```python
from build123d import *

# Parameters (mm, degrees)
F2_W      = 90
F2_H      = 90
F6_W      = 82
F6_H      = 82
F12_DEPTH = 5
F13_DEPTH = 10.1
F14_DEPTH = 10
F15_DEPTH = 10
F16_W     = 1.180001
F16_H     = 1.870001
F16_W_2   = 1.18
F16_H_2   = 4.060001
F16_W_3   = 10.110001
F16_H_3   = 1.18
F16_W_4   = 6.670001
F17_DEPTH = 2


# Not quite as in the source:
# - the dataset's text gives a spline's control points without its knots; the knots are read off the source's solid


with BuildPart() as f3:
    # F2 (on Top) → F3 section 0
    with BuildSketch(Plane.XY, mode=Mode.PRIVATE) as f3_s0:
        Rectangle(F2_W, F2_H)
    loft([f3_s0.sketch, Vertex(0, 0, 63.6368)])

    # F6 (on face) → F7 section 0
    with BuildSketch(Plane.XY, mode=Mode.PRIVATE) as f7_s0:
        Rectangle(F6_W, F6_H)
    loft([f7_s0.sketch, Vertex(0, 0, 58.6368)], mode=Mode.SUBTRACT)

    # F8 (on face) → F12 (cut, symmetric)
    with BuildSketch(Plane(origin=(29.9991167733, 0, 21.2135156827), x_dir=(0, 1, 0), z_dir=(0.8164845616, 0, 0.5773672666))):
        Polygon((0.1463476627, 39.9593571873), (-28.0024763197, -8.9000007138), (27.9615262598, -8.9000007138), align=None)
    extrude(amount=F12_DEPTH, both=True, mode=Mode.SUBTRACT)

    # F9 (on face) → F13 (cut)
    with BuildSketch(Plane(origin=(0, 29.9991167733, 21.2135156827), x_dir=(-1, 0, 0), z_dir=(0, 0.8164845616, 0.5773672666))):
        Polygon((0.1463476627, 39.9593571873), (-27.835653627, -8.5054690465), (28.1283489525, -8.5054690465), align=None)
    extrude(amount=-F13_DEPTH, mode=Mode.SUBTRACT)

    # F10 (on face) → F14 (cut)
    with BuildSketch(Plane(origin=(-29.9991167733, 0, 21.2135156827), x_dir=(0, -1, 0), z_dir=(-0.8164845616, 0, 0.5773672666))):
        Polygon((0.1463476627, 39.9593571873), (-28.9770383388, -9.5114903525), (26.9869642407, -9.5114903525), align=None)
    extrude(amount=-F14_DEPTH, mode=Mode.SUBTRACT)

    # F11 (on face) → F15 (cut)
    with BuildSketch(Plane(origin=(0, -29.9991167733, 21.2135156827), x_dir=(1, 0, 0), z_dir=(0, -0.8164845616, 0.5773672666))):
        Polygon((0.1463476627, 39.9593571873), (-28.0361250043, -9.3999961391), (27.9278775752, -9.3999961391), align=None)
    extrude(amount=-F15_DEPTH, mode=Mode.SUBTRACT)

    # F16 (on face) → F17 (cut)
    with BuildSketch(Plane(origin=(-29.9991167733, 0, 21.2135156827), x_dir=(0, -1, 0), z_dir=(-0.8164845616, 0, 0.5773672666))):
        Polygon((21.9697801374, -21.1938021154), (23.5597841374, -21.1938021154), (28.7397811374, -15.0950853876), (28.7397811374, -19.0038021154), (29.9197811374, -19.0038021154), (29.9197811374, -14.9538011154), (28.8597821374, -14.9538011154), (28.7397811374, -14.9538011154), (22.2197811374, -14.9538011154), (21.2197821374, -16.1338011154), (26.2597841374, -16.1338011154), align=None)
        with Locations((31.4797826374, -18.0688016154)):
            Rectangle(F16_W, F16_H)
        with Locations((33.6297791374, -19.1638016154)):
            Rectangle(F16_W_2, F16_H_2)
        Polygon((12.0897811374, -21.1938021154), (20.2597801374, -21.1938021154), (20.8297821374, -20.0438011154), (18.3297821374, -14.9538011154), (13.9597791374, -14.9538011154), (11.4997811374, -19.9838021154), align=None)
        Polygon((19.3697831374, -20.0138021154), (12.9197831374, -20.0138021154), (14.8197791374, -16.1338011154), (17.4797821374, -16.1338011154), align=None, mode=Mode.SUBTRACT)
        with BuildLine():
            Line((5.2997801374, -14.9538011154), (5.2997801374, -16.6038011154))
            add(Edge.make_bspline(
                [(4.1407171374, -16.7288011154), (4.3252931374, -16.7141861154), (4.7128221374, -16.6835011154), (5.0980381374, -16.6311951154), (5.2997801374, -16.6038011154)],
                knots=[0, 0, 0, 0, 0.555346, 1.165986, 1.165986, 1.165986, 1.165986], degree=3))
            add(Edge.make_bspline(
                [(3.2325931374, -16.7738011154), (3.3718421374, -16.7690131154), (3.6747741374, -16.7585981154), (3.9772701374, -16.7392531154), (4.1407171374, -16.7288011154)],
                knots=[0, 0, 0, 0, 0.417971, 0.909282, 0.909282, 0.909282, 0.909282], degree=3))
            add(Edge.make_bspline(
                [(2.4297801374, -16.7638011154), (2.5552081374, -16.7691171154), (2.8227031374, -16.7804551154), (3.0904121374, -16.7761091154), (3.2325931374, -16.7738011154)],
                knots=[0, 0, 0, 0, 0.376537, 0.803027, 0.803027, 0.803027, 0.803027], degree=3))
            Line((2.4297801374, -16.7638011154), (1.2497801374, -16.7638011154))
            Line((1.2497801374, -16.7638011154), (1.2497801374, -21.1938021154))
            Line((1.2497801374, -21.1938021154), (10.6597801374, -21.1938021154))
            Line((10.6597801374, -21.1938021154), (10.6597801374, -20.0138021154))
            Line((10.6597801374, -20.0138021154), (6.4797801374, -20.0138021154))
            Line((6.4797801374, -20.0138021154), (6.4797801374, -17.6491141154))
            add(Edge.make_bspline(
                [(8.6047791374, -17.0530201154), (8.2523501374, -17.1763541154), (7.5565571374, -17.4198491154), (6.8355751374, -17.5733591154), (6.4797801374, -17.6491141154)],
                knots=[0, 0, 0, 0, 1.118887, 2.208999, 2.208999, 2.208999, 2.208999], degree=3))
            add(Edge.make_bspline(
                [(10.6597801374, -16.1361451154), (10.3259741374, -16.3048751154), (9.6557671374, -16.6436461154), (8.9560111374, -16.9162101154), (8.6047791374, -17.0530201154)],
                knots=[0, 0, 0, 0, 1.121359, 2.251432, 2.251432, 2.251432, 2.251432], degree=3))
            Line((10.6597801374, -16.1361451154), (10.6597801374, -14.9538011154))
            add(Edge.make_bspline(
                [(8.5247801374, -15.8638011154), (8.8834781374, -15.7390181154), (9.6157961374, -15.4842611154), (10.3070901374, -15.1330071154), (10.6597801374, -14.9538011154)],
                knots=[0, 0, 0, 0, 1.137935, 2.323212, 2.323212, 2.323212, 2.323212], degree=3))
            add(Edge.make_bspline(
                [(6.4797801374, -16.4038011154), (6.8146711374, -16.3298001154), (7.5036441374, -16.1775551154), (8.1781381374, -15.9703101154), (8.5247801374, -15.8638011154)],
                knots=[0, 0, 0, 0, 1.028459, 2.115858, 2.115858, 2.115858, 2.115858], degree=3))
            Line((6.4797801374, -16.4038011154), (6.4797801374, -14.9538011154))
            Line((6.4797801374, -14.9538011154), (5.2997801374, -14.9538011154))
        make_face()
        with BuildLine():
            Line((5.2997801374, -20.0138021154), (2.4297801374, -20.0138021154))
            Line((2.4297801374, -20.0138021154), (2.4297801374, -17.9538021154))
            add(Edge.make_bspline(
                [(3.2525921374, -17.9638011154), (3.1087451374, -17.9660571154), (2.8343741374, -17.9703591154), (2.5602071374, -17.9591391154), (2.4297801374, -17.9538021154)],
                knots=[0, 0, 0, 0, 0.431492, 0.823018, 0.823018, 0.823018, 0.823018], degree=3))
            add(Edge.make_bspline(
                [(4.1557951374, -17.9288011154), (3.9935791374, -17.9363501154), (3.6926011374, -17.9503551154), (3.3914391374, -17.9595581154), (3.2525921374, -17.9638011154)],
                knots=[0, 0, 0, 0, 0.487164, 0.903894, 0.903894, 0.903894, 0.903894], degree=3))
            add(Edge.make_bspline(
                [(5.2997801374, -17.8238011154), (5.1009381374, -17.8479581154), (4.7206281374, -17.8941601154), (4.3382501374, -17.9176111154), (4.1557951374, -17.9288011154)],
                knots=[0, 0, 0, 0, 0.600755, 1.14902, 1.14902, 1.14902, 1.14902], degree=3))
            Line((5.2997801374, -17.8238011154), (5.2997801374, -20.0138021154))
        make_face(mode=Mode.SUBTRACT)
        Polygon((-7.2802218626, -14.9538011154), (-9.6202208626, -19.7238021154), (-11.9602208626, -14.9538011154), (-13.3902208626, -14.9538011154), (-10.3302198626, -21.1938021154), (-8.9002208626, -21.1938021154), (-6.4202218626, -16.1338011154), (-5.8402208626, -16.1338011154), (-5.8402208626, -21.1938021154), (-4.6602208626, -21.1938021154), (-4.6602208626, -16.1338011154), (-3.9402198626, -16.1338011154), (-3.9402198626, -14.9538011154), align=None)
        with Locations((-18.7952213626, -15.5438011154)):
            Rectangle(F16_W_3, F16_H_3)
        with Locations((-18.7952213626, -18.0738011154)):
            Rectangle(F16_W_4, F16_H_3)
        with Locations((-18.7952213626, -20.6038021154)):
            Rectangle(F16_W_3, F16_H_3)
        Polygon((-33.1302218626, -18.0738021154), (-30.4802218626, -21.1938021154), (-27.3102218626, -21.1938021154), (-24.6602208626, -18.0738021154), (-26.2502218626, -18.0738021154), (-28.3002218626, -20.4938021154), (-28.3002218626, -14.9538011154), (-29.4802218626, -14.9538011154), (-29.4802218626, -20.4938021154), (-31.5402218626, -18.0738021154), align=None)
    extrude(amount=-F17_DEPTH, mode=Mode.SUBTRACT)


solid = f3.part
```
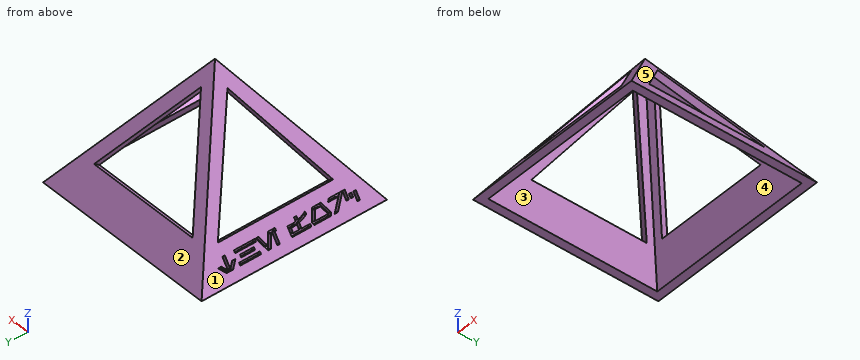
Model file for the job. Use its own axes, mm. Face numbers are marked on the shaded views. A direction names the side the tool comes from. Give positions to 0.01 mm unless a question says otherwise; leave off trailing zeros. Write each loop counter-clockwise with the first axis right and the second up, starting at its lowest first coordinate (ties: lowest second). Pieces come first, ordered by that corner, then holes. Notation, with made-up numbers: (13, 86) -> (21, 86) arc R27 ccw to (21, 121) -> close; hole circle Ø8 at (84, 35). An arc over 180 degrees is marked (long way). Use CSV: the item, a comma, the result in double quotes. Start each with the question number.
1) Two-plate mould, pull along Y, no slides. Class the marked faces 1, 2 and 3: released by +Y, released by -Y, zero draft, split by the parting line, or undercut.
2) Cut at D-D on y = 2. List the corners of the cut face in (x, z) (1 decimal).
3) Cut at A-A on x = 21. List the corners of the cut face in (y, z).
4) Cut at B-B on z = 19.5. List the corners of the cut face in (x, y).
5) Pin check, flat tips, straight feed: P1, Ø3, axis at x = -38, z = 8, coming from the -Y side; P2, Ø2.5, axis at x = -40, z = 6.5, coming from the +Y side; P3, Ø1.2, axis at x = -38.5, z = 7, coming from the -Y side. Stop position of each tip, or through.
6) Tool access for the marked faces 4 and 5: list every direction of +Z, -Z, +X, -X, +Y, -Y with a clear straight run to the whole face (end or side of a thin tool).
7) Cut at C-C on y = 19.5. Count the separate pieces of the cut face and the enclosed holes in it, plus the area to 3 significant figures.
8) Drill centre lines: L1, parallel to Y at x = -24.5, z = 13; L2, parallel to Y at x = -8, z = 4; L3, parallel to X at y = -32, z = 9.5. Where is each one in solid material? Low to high.
Final values:
1,face 1,"zero draft"
1,face 2,"released by +Y"
1,face 3,"undercut"
2,outline,"(-45, 0) -> (-41, 0) -> (-32.9, 11.6) -> (-35.5, 13.4) -> close; (-9, 50.9) -> (-6.6, 49.2) -> (-2, 55.8) -> (2, 55.8) -> (6.4, 49.5) -> (8.8, 51.2) -> (2, 60.8) -> (-2, 60.8) -> close; (32.5, 12.1) -> (41, 0) -> (45, 0) -> (35.1, 13.9) -> close"
3,outline,"(-45, 0) -> (-41, 0) -> (-32.82, 11.7) -> (-35.43, 13.54) -> close; (-28.32, 23.59) -> (-25.77, 21.78) -> (-21, 28.6) -> (-16.41, 28.6) -> (-13.9, 33.94) -> (-21, 33.94) -> close; (14.02, 33.94) -> (16.5, 28.6) -> (21, 28.6) -> (25.52, 22.13) -> (28.07, 23.94) -> (21, 33.94) -> close; (32.31, 12.43) -> (41, 0) -> (45, 0) -> (34.91, 14.27) -> close"
4,outline,"(-31.21, -31.21) -> (-23.87, -31.21) -> (-22.6, -27.37) -> (-27.37, -27.37) -> (-27.37, -21.76) -> (-31.21, -22.97) -> close; (-31.21, 24.61) -> (-27.37, 23.31) -> (-27.37, 27.37) -> (-23.15, 27.37) -> (-24.43, 31.21) -> (-31.21, 31.21) -> close; (22.57, -27.37) -> (23.82, -31.21) -> (31.21, -31.21) -> (31.21, -24.08) -> (27.37, -22.8) -> (27.37, -27.37) -> close; (22.85, 27.37) -> (27.37, 27.37) -> (27.37, 22.83) -> (31.21, 24.09) -> (31.21, 31.21) -> (24.14, 31.21) -> close"
5,P1,"stops at y = -40.4"
5,P2,"stops at y = 41.29"
5,P3,"stops at y = -40.47"
6,face 4,"-Z"
6,face 5,"+Z, +X, +Y, -Y"
7,separate pieces,"4"
7,enclosed holes,"0"
7,area,"214 mm2"
8,L1,"y = -35.81 to -34.66, 33.12 to 35.81"
8,L2,"y = -42.17 to -38.2, 38.2 to 42.17"
8,L3,"x = -38.28 to -34.36, 34.36 to 38.28"
